The model under review builds one solid part; all positions refer to its coordinate system, in mm. Face numbers are marked on the shaded views. A direction names the side the tool comes from. Coordinates: 2 decimals unless noted, no trailing zeros. Write each loop counter-clockwise with the first axis right and the second up, starting at its lowest first coordinate (ties: lowest second). Pieces come first, ordered by that corner, then holes.
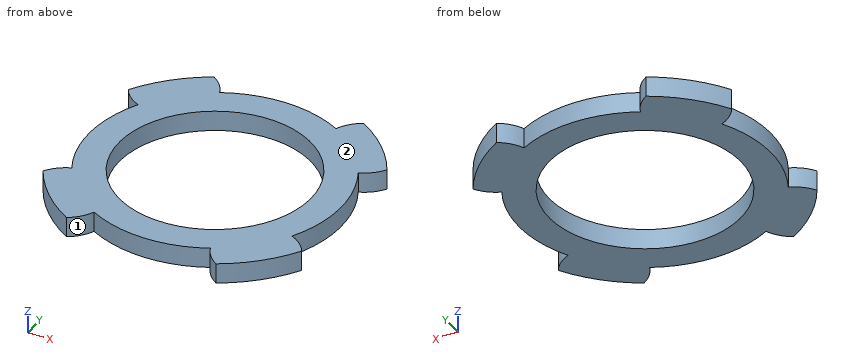
```python
from build123d import *
from build123d.topology import SkipClean

# Parameters (mm, degrees)
SKETCH3_R             = 4
BOSS_EXTRUDE1_DEPTH   = 11
BOSS_EXTRUDE1_2_DEPTH = 11
BOSS_EXTRUDE1_3_DEPTH = 11
BOSS_EXTRUDE1_4_DEPTH = 11
BOSS_EXTRUDE6_START   = 2
SKETCH6_R             = 9.5
BOSS_EXTRUDE6_DEPTH   = 2
SKETCH7_R             = 19.191160133
CUT_EXTRUDE1_DEPTH    = 11


with BuildPart() as part:
    # Sketch3 → Boss-Extrude1 (new body)
    with BuildSketch(Plane(origin=(0, 0, 15), x_dir=(-1, 0, 0), z_dir=(0, 0, -1))):
        with Locations((-9.545941546, 9.545941546)):
            Circle(SKETCH3_R)
    extrude(amount=BOSS_EXTRUDE1_DEPTH)



with BuildPart() as body_2:
    # Sketch3 → Boss-Extrude1 2 (new body)
    with BuildSketch(Plane(origin=(0, 0, 15), x_dir=(-1, 0, 0), z_dir=(0, 0, -1))):
        with Locations((9.545941546, 9.545941546)):
            Circle(SKETCH3_R)
    extrude(amount=BOSS_EXTRUDE1_2_DEPTH)


with BuildPart() as body_3:
    # Sketch3 → Boss-Extrude1 3 (new body)
    with BuildSketch(Plane(origin=(0, 0, 15), x_dir=(-1, 0, 0), z_dir=(0, 0, -1))):
        with Locations((9.545941546, -9.545941546)):
            Circle(SKETCH3_R)
    extrude(amount=BOSS_EXTRUDE1_3_DEPTH)


with BuildPart() as body_4:
    # Sketch3 → Boss-Extrude1 4 (new body)
    with BuildSketch(Plane(origin=(0, 0, 15), x_dir=(-1, 0, 0), z_dir=(0, 0, -1))):
        with Locations((-9.545941546, -9.545941546)):
            Circle(SKETCH3_R)
    extrude(amount=BOSS_EXTRUDE1_4_DEPTH)


with BuildPart() as part_1:
    with SkipClean():  # the faces are left unmerged after this step: merging them gives an invalid solid
        add(part.part)

        add(body_2.part)  # Boss-Extrude6 merges body 2

        add(body_3.part)  # Boss-Extrude6 merges body 3

        add(body_4.part)  # Boss-Extrude6 merges body 4
        # Sketch6 → Boss-Extrude6 (add)
        with BuildSketch(Plane.XY.offset(15).offset(BOSS_EXTRUDE6_START)):
            with BuildLine():
                ThreePointArc((-5.840211131, 11.051784197), (-6.514660932, 12.155795534), (-7.506206096, 12.986795988))
                ThreePointArc((-7.506206096, 12.986795988), (-10.606601718, 10.606601718), (-12.986795988, 7.506206096))
                ThreePointArc((-12.986795988, 7.506206096), (-12.155795534, 6.514660932), (-11.051784197, 5.840211131))
                ThreePointArc((-11.051784197, 5.840211131), (-12.5, 0), (-11.051784197, -5.840211131))
                ThreePointArc((-11.051784197, -5.840211131), (-12.155795534, -6.514660932), (-12.986795988, -7.506206096))
                ThreePointArc((-12.986795988, -7.506206096), (-10.606601718, -10.606601718), (-7.506206096, -12.986795988))
                ThreePointArc((-7.506206096, -12.986795988), (-6.514660932, -12.155795534), (-5.840211131, -11.051784197))
                ThreePointArc((-5.840211131, -11.051784197), (0, -12.5), (5.840211131, -11.051784197))
                ThreePointArc((5.840211131, -11.051784197), (6.514660932, -12.155795534), (7.506206096, -12.986795988))
                ThreePointArc((7.506206096, -12.986795988), (10.606601718, -10.606601718), (12.986795988, -7.506206096))
                ThreePointArc((12.986795988, -7.506206096), (12.155795534, -6.514660932), (11.051784197, -5.840211131))
                ThreePointArc((11.051784197, -5.840211131), (12.5, 0), (11.051784197, 5.840211131))
                ThreePointArc((11.051784197, 5.840211131), (12.155795534, 6.514660932), (12.986795988, 7.506206096))
                ThreePointArc((12.986795988, 7.506206096), (10.606601718, 10.606601718), (7.506206096, 12.986795988))
                ThreePointArc((7.506206096, 12.986795988), (6.514660932, 12.155795534), (5.840211131, 11.051784197))
                ThreePointArc((5.840211131, 11.051784197), (0, 12.5), (-5.840211131, 11.051784197))
            make_face()
            Circle(SKETCH6_R, mode=Mode.SUBTRACT)
        extrude(amount=-BOSS_EXTRUDE6_DEPTH)

    # Sketch7 → Cut-Extrude1 (cut)
    with BuildSketch(Plane(origin=(0, 0, 4), x_dir=(-1, 0, 0), z_dir=(0, 0, -1))):
        Circle(SKETCH7_R)
    extrude(amount=-CUT_EXTRUDE1_DEPTH, mode=Mode.SUBTRACT)


solid = part_1.part
```
Item 1: To check wall thickness, follow line 1 along Y through (x, z) = (0, 15.9); line 2 along X through (y, z) = (-5.5, 15.15); line 3 along X through (y, z) = (-4, 15.1). State the ranges of each line that lie inside material, in increasing order.
Solved:
line 1: y = -12.5 to -9.5, 9.5 to 12.5
line 2: x = -11.22 to -7.75, 7.75 to 11.22
line 3: x = -11.84 to -8.62, 8.62 to 11.84
Item 2: Machinability: for the marked faces 1 and 2, which of the approach directions +Z, -Z, +X, -X, +Y, -Y give a long, thin tool a straight path to every point of the face, cutting with its end or side? Answer none if there is none.
Solved:
face 1: +Z, -Z, -Y
face 2: +Z, +X, -X, +Y, -Y
Item 3: Take a section at B-B, the plane z = 16.1. Write out the cut boundary in (x, y), plus the area to 3 significant figures.
Solved:
outline: (-12.99, -7.51) arc R15 ccw to (-7.51, -12.99) arc R4 ccw to (-5.84, -11.05) arc R12.5 ccw to (5.84, -11.05) arc R4 ccw to (7.51, -12.99) arc R15 ccw to (12.99, -7.51) arc R4 ccw to (11.05, -5.84) arc R12.5 ccw to (11.05, 5.84) arc R4 ccw to (12.99, 7.51) arc R15 ccw to (7.51, 12.99) arc R4 ccw to (5.84, 11.05) arc R12.5 ccw to (-5.84, 11.05) arc R4 ccw to (-7.51, 12.99) arc R15 ccw to (-12.99, 7.51) arc R4 ccw to (-11.05, 5.84) arc R12.5 ccw to (-11.05, -5.84) arc R4 ccw to start; hole circle Ø19 at (0, 0)
area: 287 mm2
Item 4: Take a section at A-A, the plane y = 0. Write out the cut boundary in (x, z).
Solved:
outline: (-12.5, 15) - (-9.5, 15) - (-9.5, 17) - (-12.5, 17) - close; (9.5, 15) - (12.5, 15) - (12.5, 17) - (9.5, 17) - close
Item 5: Take a section at D-D, the plane x = -10.5. Write out the cut boundary in (y, z), plus the area to 3 significant figures.
Solved:
outline: (-10.71, 15) - (10.71, 15) - (10.71, 17) - (-10.71, 17) - close
area: 42.8 mm2
